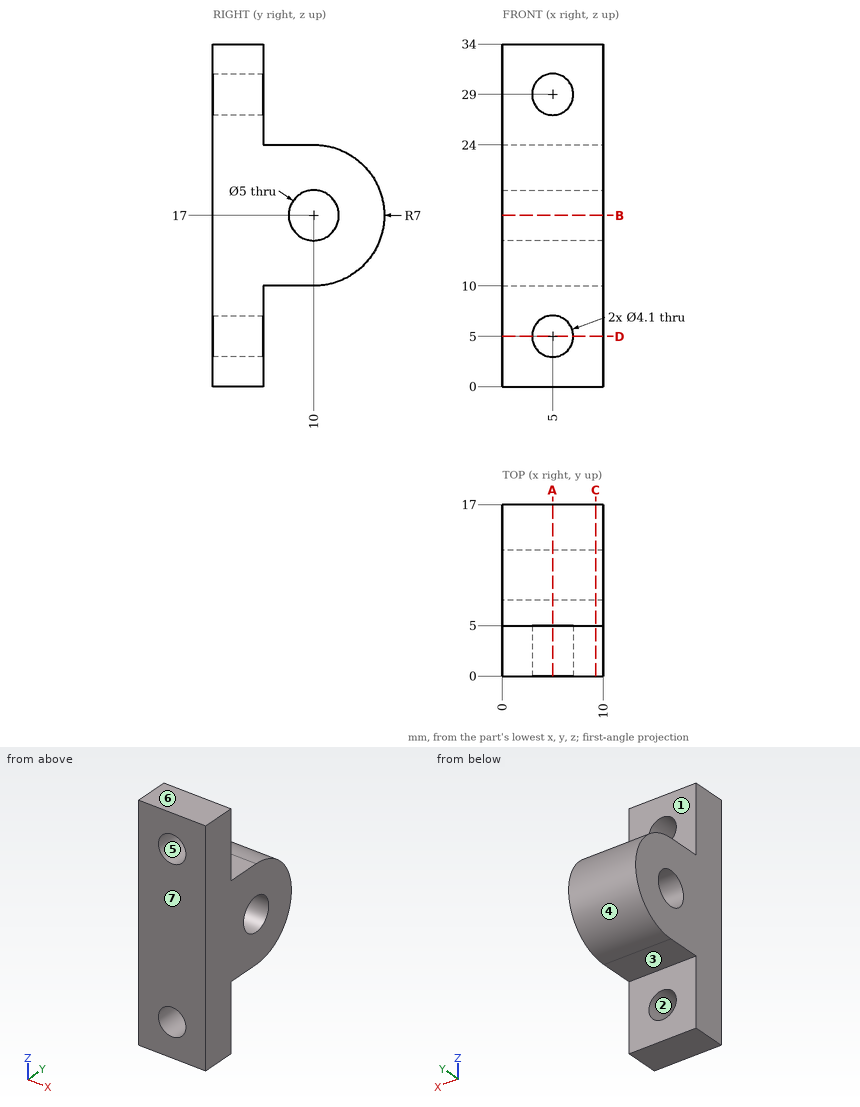
Check sheet for the drawn part. Datum: minimum x, y, z corner. Units: mm. A direction names the side the tool comes from. Coordinates: 2 decimals unless noted, no trailing zeros. Order: outer loops, then holes, each group sorted by start corner. A loop starts at its lowest first (then second) coordinate and runs counter-clockwise, first axis right, second up. Notation, with made-up numbers: (-24.5, 60.5) - (-6.5, 60.5) arc R21 cw to (-6.5, 73.5) - close; hole circle Ø8 at (65, 57.5). An arc over 180 degrees is marked (long way). Return JSON: item names as keys, results as strings.
(1) Mould release check, pull along Z, two halves, no side actions. Record for the marked faces 4, 5, 6 and 7: pulls with the +Z half, pulls with the -Z half, needs draft (parallel to the pull), parting line crosses it, or undercut.
Filled sheet:
{"face 4": "parting line crosses it", "face 5": "undercut", "face 6": "pulls with the +Z half", "face 7": "needs draft"}
(2) Section check C-C, the plane x = 9.25. Record the cut outline in (y, z), and give its area (3 significant figures).
Filled sheet:
{"outline": "(0, 0) - (5, 0) - (5, 10) - (10, 10) arc R7 ccw to (10, 24) - (5, 24) - (5, 34) - (0, 34) - close; hole circle Ø5 at (10, 17)", "area": "297 mm^2"}
(3) Thickness scan on line 1 along Z through (x, y) = (3.25, 10); line 2 along Y through (x, z) = (6.5, 17); line 3 along X through (y, z) = (3.5, 5). Record the ranges inside material, lowest first.
Filled sheet:
{"line 1": "z = 10 to 14.5, 19.5 to 24", "line 2": "y = 0 to 7.5, 12.5 to 17", "line 3": "x = 0 to 2.95, 7.05 to 10"}
(4) Go/stop test with flat-tipped pins: pin 1 (2.5 mm diameter, centred on x = 5.5, y = 8.5, fed in from -Z); pin 2 (1.5 mm diameter, centred on x = 6, z = 7, fed in from +Y); pin 3 (3.5 mm diameter, centred on x = 5, z = 29, fed in from +Y); pin 4 (2.5 mm diameter, centred on x = 5, y = 7.5, fed in from +Z). Record where each tip stops, or that it passes through.
Filled sheet:
{"pin 1": "stops at z = 10", "pin 2": "stops at y = 5", "pin 3": "passes through", "pin 4": "stops at z = 24"}
(5) Access from +Z, -Z, +X, -X, +Y, -Y to the whole of each face (thin tool, end or side, straight path). Record for the marked faces 1, 2 and 3.
Filled sheet:
{"face 1": "+Z, +X, -X, +Y", "face 2": "+Y, -Y", "face 3": "-Z, +X, -X, +Y"}
(6) Section check B-B, the plane z = 17. Record the cut outline in (x, y), and give its area (3 significant figures).
Filled sheet:
{"outline": "(0, 0) - (10, 0) - (10, 7.5) - (0, 7.5) - close; (0, 12.5) - (10, 12.5) - (10, 17) - (0, 17) - close", "area": "120 mm^2"}
(7) Section check A-A, the plane x = 5. Record the cut outline in (y, z).
Filled sheet:
{"outline": "(0, 0) - (5, 0) - (5, 2.95) - (0, 2.95) - close; (0, 7.05) - (5, 7.05) - (5, 10) - (10, 10) arc R7 ccw to (10, 24) - (5, 24) - (5, 26.95) - (0, 26.95) - close; (0, 31.05) - (5, 31.05) - (5, 34) - (0, 34) - close; hole circle Ø5 at (10, 17)"}
(8) Section check D-D, the plane z = 5. Record the cut outline in (x, y), and give its area (3 significant figures).
Filled sheet:
{"outline": "(0, 0) - (2.95, 0) - (2.95, 5) - (0, 5) - close; (7.05, 0) - (10, 0) - (10, 5) - (7.05, 5) - close", "area": "29.5 mm^2"}
